Source: three-view drawing plus pictorial views. Frame: mm from the lowest corner of the part. A direction names the side the tool comes from. Coordinates: 2 decimals unless noted, no trailing zeros. Write each loop counter-clockwise with the first axis right and the second up, starting at its lowest first coordinate (ties: lowest second). Pieces come first, ordered by that corner, then holes. Notation, with made-up numbers: (10.25, 69.5) - (64.25, 69.5) arc R17 cw to (64.25, 87.5) - close; hole circle Ø11 at (19, 83.5). An arc over 180 degrees is marked (long way). Put each result on its own line as item: value.
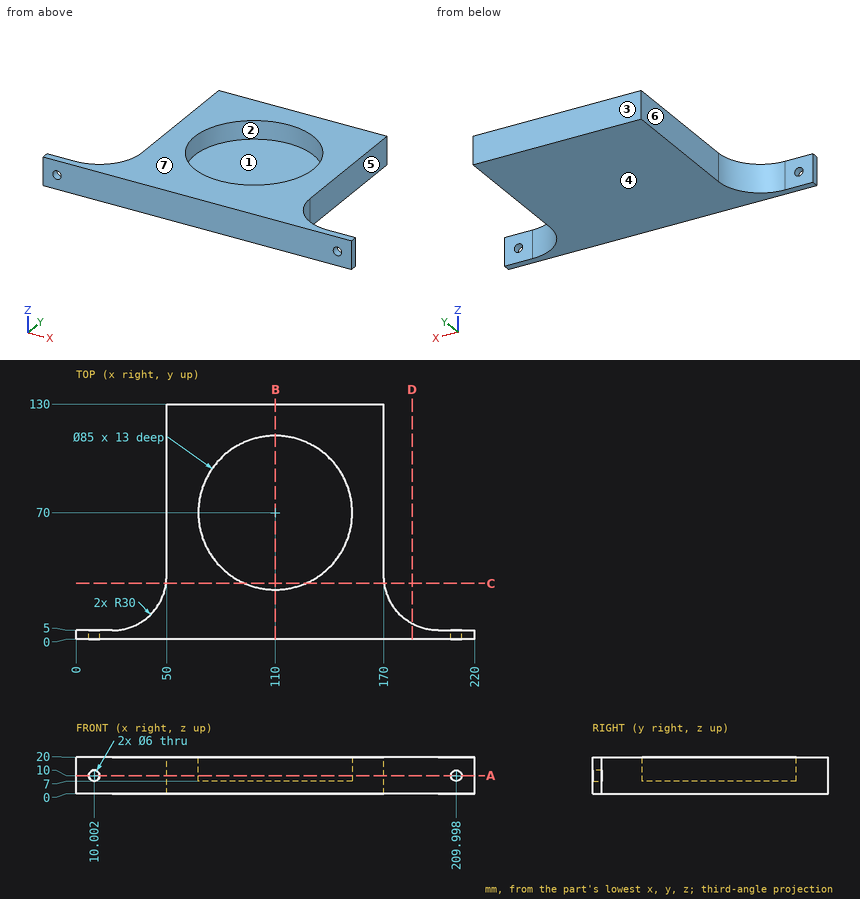
1. Section query D-D (x = 185.5). Return loops of the section in (y, z).
Answer below:
outline: (0, 0) - (8.74, 0) - (8.74, 20) - (0, 20) - close
2. Pin query (flat end, axial travel): pin 1 Ø6 at (x, z) = (205.5, 12.5) entering from +Y; pin 2 Ø3.5 at (x, z) = (10, 10) entering from +Y; pin 3 Ø2 at (y, z) = (70, 15) entering from +X. Return the tip coordinate at first contact, or that it passes through.
Answer below:
pin 1: stops at y = 5
pin 2: passes through
pin 3: stops at x = 170
3. Mould query, pull axis Y, two halves, no side actions, for the marked faces 1, 2, 3 and 4. Classes: +Y half, -Y half, draft (parallel to the pull), parting line (faces both ways), or undercut.
Answer below:
face 1: undercut
face 2: undercut
face 3: +Y half
face 4: draft
4. Set-up query: the marked faces 5, 6 and 7. Return all of +Z, -Z, +X, -X, +Y, -Y with unobstructed straight access to the full face (end or side cutting, diameter ignored); none if empty.
Answer below:
face 5: +Z, -Z, +X, +Y
face 6: +Z, -Z, -X, +Y
face 7: +Z, +X, -X, +Y, -Y
5. Ray query, probe 1 along X at (y, z) = (3.4, 10); probe 2 along X at (y, z) = (68.5, 13.75); probe 3 along X at (y, z) = (50.5, 3.25). Return the intervals inside material, ascending. Write a range as from..to.
Answer below:
probe 1: x = 0..7, 13..207, 213..220
probe 2: x = 50..67.53, 152.47..170
probe 3: x = 50..170
6. Section query B-B (x = 110). Return loops of the section in (y, z), then the cut area to 4 significant figures.
Answer below:
outline: (0, 0) - (130, 0) - (130, 20) - (112.5, 20) - (112.5, 7) - (27.5, 7) - (27.5, 20) - (0, 20) - close
area: 1,495 mm²
7. Section query A-A (z = 10). Return loops of the section in (x, y).
Answer below:
outline: (0, 0) - (7, 0) - (7, 5) - (0, 5) - close; (13, 0) - (207, 0) - (207, 5) - (200, 5) arc R30 cw to (170, 35) - (170, 130) - (50, 130) - (50, 35) arc R30 cw to (20, 5) - (13, 5) - close; (213, 0) - (220, 0) - (220, 5) - (213, 5) - close; hole circle Ø85 at (110, 70)
8. Section query C-C (y = 31). Return loops of the section in (x, z), then the cut area to 3 significant figures.
Answer below:
outline: (49.73, 0) - (170.27, 0) - (170.27, 20) - (126.89, 20) - (126.89, 7) - (93.11, 7) - (93.11, 20) - (49.73, 20) - close
area: 1,970 mm²
